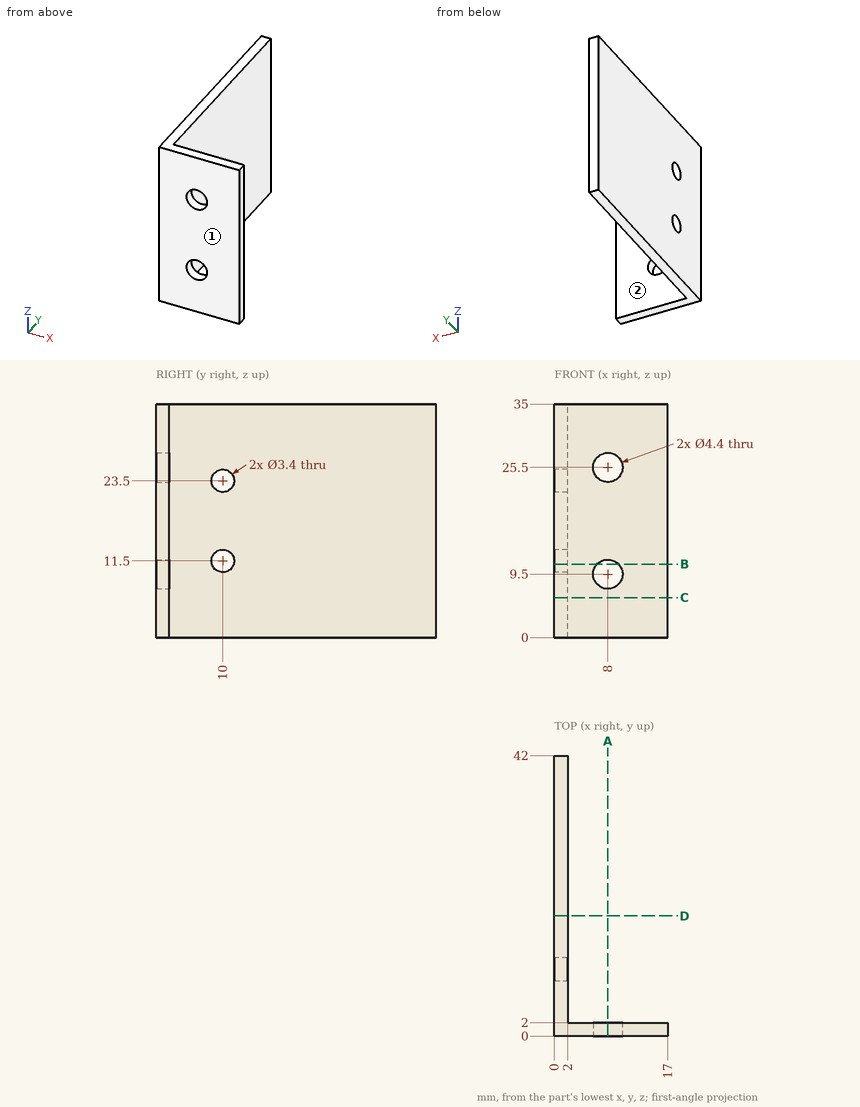
The figure shows three views and two pictorial views of one solid part (mm, origin at its lowest corner). Answer the questions. A direction names the side the tool comes from. Give positions to 0.01 mm unless a question says otherwise; leave off trailing zeros. Order: outer loops, then holes, each group sorted by start corner. A loop starts at its lowest first (then second) coordinate and runs counter-clockwise, first axis right, second up. Notation, with made-up numbers: M -23,24.25 L -19,24.25 A18 ccw -19,29.25 Z; hole C 31.25,-31 d4. An arc over 180 degrees is marked long. Return JSON: item names as keys, results as strings.
1) Section A-A, the plane x = 8 is taken. Write down the section's boundary in (y, z).
Resolved:
{"outline": "M 0,0 L 2,0 L 2,7.3 L 0,7.3 Z; M 0,11.7 L 2,11.7 L 2,23.3 L 0,23.3 Z; M 0,27.7 L 2,27.7 L 2,35 L 0,35 Z"}
2) Each of these flat-tipped pins is pushed along its axis until it touches: pin 1 (4 mm diameter, centred on x = 8, z = 9.5, fed in from -Y); pin 2 (1 mm diameter, centred on y = 33, z = 26, fed in from +X); pin 3 (2 mm diameter, centred on x = 14.5, z = 14, fed in from -Y); pin 4 (2 mm diameter, centred on x = 10.5, z = 18.5, fed in from +Y). Where does it stop, or does it pass through?
Resolved:
{"pin 1": "through", "pin 2": "x = 2", "pin 3": "y = 0", "pin 4": "y = 2"}
3) Section C-C, the plane z = 6 is taken. Write down the section's boundary in (x, y), plus the area to 3 significant figures.
Resolved:
{"outline": "M 0,0 L 17,0 L 17,2 L 2,2 L 2,42 L 0,42 Z", "area": "114 mm^2"}
4) Straight lines are drawn through the part: line 1 along Z through (x, y) = (0.75, 10); line 2 along Z through (x, y) = (8, 0.6); line 3 along Y through (x, z) = (15, 5). For each, find the intervals that lie inside material, in ascending order. Write a range as [from, to].
Resolved:
{"line 1": "[0, 9.8], [13.2, 21.8], [25.2, 35]", "line 2": "[0, 7.3], [11.7, 23.3], [27.7, 35]", "line 3": "[0, 2]"}
5) Section D-D, the plane y = 18 is taken. Write down the section's boundary in (x, z), plus the area to 3 significant figures.
Resolved:
{"outline": "M 0,0 L 2,0 L 2,35 L 0,35 Z", "area": "70.0 mm^2"}
6) A tool of negligible diameter and unlimited length cuts with its end or side. For the marked faces 1 and 2, from which of +Z, -Z, +X, -X, +Y, -Y can it reach the whole face along a straight path? Write none if from no direction.
Resolved:
{"face 1": "+Z, -Z, +X, -X, -Y", "face 2": "+Z, -Z, +X, +Y"}
7) Section B-B, the plane z = 11 is taken. Write down the section's boundary in (x, y).
Resolved:
{"outline": "M 0,0 L 6.39,0 L 6.39,2 L 2,2 L 2,8.38 L 0,8.38 Z; M 0,11.62 L 2,11.62 L 2,42 L 0,42 Z; M 9.61,0 L 17,0 L 17,2 L 9.61,2 Z"}
